from build123d import *

# Parameters (mm, degrees)
SKETCH1_R            = 1.5
BOSS_EXTRUDE1_DEPTH  = 3
SKETCH3_R            = 1.7144
SKETCH3_R_2          = 3.2384
SKETCH3_R_3          = 3.4289
SKETCH3_R_4          = 1.714400001
CUT_EXTRUDE4_DEPTH   = 106.238487343
SKETCH4_R            = 1.5
CUT_EXTRUDE5_DEPTH   = 106.238487343
CABLEHOLE_DEPTH      = 106.238487343
CABLEHOLE_DEPTH_BACK = 106.238487343
FILLET1_R            = 5


with BuildPart() as part:
    # Sketch1 → Boss-Extrude1 (new body)
    with BuildSketch(Plane.XY):
        Polygon((9.894788559, 90.661246725), (-9.906811441, 90.661246725), (-53.35426469, 15.408050237), (-53.35426469, -15.894788559), (9.894788559, -15.894788559), align=None)
        with BuildLine():
            Line((2.984475762, -9.894788559), (2.984475762, -11.107284946))
            ThreePointArc((2.984475762, -11.107284946), (-1.404084484, -11.470508377), (-5.516079054, -9.894788559))
            Line((-5.516079054, -9.894788559), (2.984475762, -9.894788559))
        make_face(mode=Mode.SUBTRACT)
        with BuildLine():
            Line((-42.353698644, -10.344103475), (-42.353698644, -9.894788559))
            Line((-42.353698644, -9.894788559), (-29.988741988, -9.894788559))
            Line((-29.988741988, -9.894788559), (-29.988741988, -12.894788559))
            Line((-29.988741988, -12.894788559), (-42.353698644, -12.894788559))
            Line((-42.353698644, -12.894788559), (-42.353698644, -12.445473643))
            ThreePointArc((-42.353698644, -12.445473643), (-42.783156326, -11.394788559), (-42.353698644, -10.344103475))
        make_face(mode=Mode.SUBTRACT)
        with Locations((-19.684611441, -11.394788559)):
            Circle(SKETCH1_R, mode=Mode.SUBTRACT)
    extrude(amount=BOSS_EXTRUDE1_DEPTH)

    # Sketch3 → Cut-Extrude4 (cut, through all)
    with BuildSketch(Plane.XY):
        with Locations((-0.011311441, -6.275188559)):
            Circle(SKETCH3_R)
        with Locations((-0.277311441, 7.815511441)):
            Circle(SKETCH3_R_2)
        with Locations((-0.277311441, 20.515511441)):
            Circle(SKETCH3_R_2)
        with Locations((-0.277311441, 33.380511441)):
            Circle(SKETCH3_R_2)
        with Locations((-2.436311441, 48.341911441)):
            Circle(SKETCH3_R_3)
        with Locations((-0.011311441, 58.266061441)):
            Circle(SKETCH3_R_4)
    extrude(amount=CUT_EXTRUDE4_DEPTH, mode=Mode.SUBTRACT)

    # Sketch4 → Cut-Extrude5 (cut, through all)
    with BuildSketch(Plane.XY):
        with Locations((-42.651822313, 24.9452242)):
            Circle(SKETCH4_R)
        with Locations((-31.151822313, 44.863808487)):
            Circle(SKETCH4_R)
        Polygon((-40.200860419, 32.190414728), (-36.200860419, 39.118617958), (-33.602784207, 37.618617958), (-37.602784207, 30.690414728), align=None)
        Polygon((-24.700860419, 59.037202245), (-28.700860419, 52.108999015), (-26.102784207, 50.608999015), (-22.102784207, 57.537202245), align=None)
        Polygon((-51.700860419, 12.271830441), (-47.700860419, 19.200033671), (-45.102784207, 17.700033671), (-49.102784207, 10.771830441), align=None)
    extrude(amount=CUT_EXTRUDE5_DEPTH, mode=Mode.SUBTRACT)

    # Sketch5 → CableHole (cut, two sides: drawn at the far end of the back side and taken through both)
    with BuildSketch(Plane.XY.offset(3).offset(-CABLEHOLE_DEPTH_BACK)):
        with BuildLine():
            Line((-35.366569483, 11.996089665), (-21.139931787, 36.637348974))
            ThreePointArc((-21.139931787, 36.637348974), (-15.361765759, 38.185603895), (-13.813510838, 32.407437867))
            Line((-13.813510838, 32.407437867), (-28.040148533, 7.766178558))
            ThreePointArc((-28.040148533, 7.766178558), (-33.818314562, 6.217923637), (-35.366569483, 11.996089665))
        make_face()
    extrude(amount=CABLEHOLE_DEPTH + CABLEHOLE_DEPTH_BACK, mode=Mode.SUBTRACT)

    # Fillet1
    fillet1_edges = [part.edges().sort_by_distance(p)[0] for p in [
        (-53.35426469, -15.894788559, 1.5),
        (-53.35426469, 15.408050237, 1.5),
        (-9.906811441, 90.661246725, 1.5),
        (9.894788559, 90.661246725, 1.5),
        (9.894788559, -15.894788559, 1.5),
    ]]
    fillet(fillet1_edges, radius=FILLET1_R)


solid = part.part
CAD build for the part. Positions are in the model's coordinates, mm. A direction names the side the tool comes from. Give positions to 0.01 mm unless a question says otherwise; leave off trailing zeros. Write each loop counter-clockwise with the first axis right and the second up, starting at its lowest first coordinate (ties: lowest second). Pieces come first, ordered by that corner, then holes. Notation, with made-up numbers: (16.25, 21) - (64.25, 21) arc R20 ccw to (64.25, 48) - close; hole circle Ø9 at (31, 72). An arc over 180 degrees is marked (long way). Put each result on its own line as item: value.
(1) Saw through at A-A (y = 28.5). List the corners of the cut face in (x, z), then the cut area to 3 significant figures.
Working result:
outline: (-45.8, 0) - (-25.84, 0) - (-25.84, 3) - (-45.8, 3) - close; (-16.07, 0) - (9.89, 0) - (9.89, 3) - (-16.07, 3) - close
area: 138 mm^2
(2) Wall check: L1, parallel to Y at x = -4.5, z = 2.1; L2, parallel to X at y = 35, z = 0.2; L3, parallel to X at y = 32, z = 1.05. Give the ranges that are in metal, low to high.
Working result:
L1: -15.89 to -10.49, -9.89 to 45.6, 51.08 to 90.66
L2: -42.04 to -38.58, -35.11 to -22.09, -13.27 to -3.08, 2.53 to 9.89
L3: -43.77 to -39.87, -36.85 to -23.82, -14.05 to -3.21, 2.65 to 9.89
(3) Pull direction X, two halves, no side cores. Call faces 1 (the cylindrical face through (-9.49, 90.01, 1.52)), 2 (the flat face through (-15, 26, 0)), 3 (the flat face through (-28.353, 24.144, 1.479)): released by +X, released by -X, zero draft, split by the parting line, or undercut.
Working result:
face 1: released by -X
face 2: zero draft
face 3: undercut
(4) Saw through at B-B (z = 0.9). Count the separate pieces of the cut face and the enclosed holes in it, then the cut area to 3 significant figures.
Working result:
separate pieces: 1
enclosed holes: 15
area: 4,490 mm^2
(5) Tool access for faces 4 (the flat face through (-22, -15.895, 1)), 5 (the flat face through (-23.384, 58.277, 1.479)): list every direction of +Z, -Z, +X, -X, +Y, -Y with a clear straight run to the whole face (end or side of a thin tool).
Working result:
face 4: +Z, -Z, +X, -X, -Y
face 5: +Z, -Z
